Autodesk Inventor part; units mm, degrees
ref_plane "YZ Plane" through (0, 0, 0) normal (1, 0, 0) x (0, 1, 0)
ref_plane "XZ Plane" through (0, 0, 0) normal (0, 1, 0) x (-1, 0, 0)
ref_plane "XY Plane" through (0, 0, 0) normal (0, 0, 1) x (1, 0, 0)
sketch "Sketch1" plane through (0, 0, 0) normal (0, 0, 1) x (1, 0, 0)
  line L0 (-127.68, 259.036) -> (-127.68, -85.275)
  line L1 (-127.68, 259.036) -> (47.477, 259.036)
  line L2 (127.68, -259.036) -> (-32.32, -259.036)
  line L3 (-32.32, -259.036) -> (-127.68, -85.275)
  line L4 (127.68, -259.036) -> (127.68, -145.836)
  line L5 (127.68, -145.836) -> (47.477, 259.036)
  point P0 (0, 0)
  dimension "d6" = 344.311
  dimension "d7" = 175.157
  dimension "d9" = 160
  dimension "d10" = 113.2
extrude "Extrusion1" add sketch "Sketch1" along normal mid plane 13
sketch "Sketch2" plane through (0, 0, 6.5) normal (0, 0, 1) x (1, 0, 0)
  circle A0 centre (-71.723, 203.108) radius 9
  circle A1 centre (-71.723, 69.5056) radius 9
  line L0 (47.477, 259.036) -> (-127.68, 259.036)
  line L1 (-127.68, 259.036) -> (-127.68, -85.275)
  circle A2 centre (-71.723, 136.306) radius 5
  point P0 (0, 0)
  dimension "d17" = 55.957
  dimension "d39" = 10
  dimension "d43" = 55.928
  dimension "d44" = 66.8004
  dimension "d45" = 66.802
extrude "Extrusion4" cut sketch "Sketch2" against normal blind 25.4
properties part number "CNC-X-axis- side plates"
Can you work these out from the model? Positions are in its coordinate system, mm. Coordinates: 2 decimals unless noted, no trailing zeros. Loops run counter-clockwise (first coordinate to the right, second up) from the corner with the lowest first, then second, coordinate; pieces in that order, holes last. Notation, with made-up numbers: M -12,26.25 L 19,26.25 A19 cw 19,56.25 Z; hole C 48,30 d6. An arc over 180 degrees is marked long. Put each result on its own line as item: value. Start each with the question number.
(1) Will these pins go through, and if not, where does the flat tip stop? pin 1 Ø1 at (y, z) = (81, -4) entering from +X; pin 2 Ø16 at (x, y) = (-71.723, 203.108) entering from -Z.
(2) We'd pull the mould along X, two halves only. Please class faces 1 (the face through (88.14, 53.77, -0.09)), 2 (the face through (49, -259.036, 0)), 3 (the face through (-72.895, 212.031, 0.091)): +X half, -X half, draft (parallel to the pull), parting line (faces both ways), or undercut.
(3) Imagine slicing it at B-B on x = -109.5. List the corners of the cut face in (y, z) for me, and give its area (3 significant figures).
(4) Imagine slicing it at A-A on z = -1.5. List the corners of the cut face in (x, y) for me (3 decimals), and give its area (3 significant figures).
(5) I need wall thicknesses on probe 1 along X at (y, z) = (135.5, 3.5); probe 2 along X at (y, z) = (63.5, -3); probe 3 along X at (y, z) = (6, -5.25). Which ranges of each line are inside material? Lowest first, please.
(6) Imagine slicing it at C-C on y = -210. List the corners of the cut face in (x, z) for me.
Worked answers:
1. pin 1: stops at x = 82.84
1. pin 2: passes through
2. face 1: +X half
2. face 2: draft
2. face 3: undercut
3. outline: M -118.4,-6.5 L 259.04,-6.5 L 259.04,6.5 L -118.4,6.5 Z
3. area: 4,910 mm2
4. outline: M -127.68,-85.275 L -32.32,-259.036 L 127.68,-259.036 L 127.68,-145.836 L 47.477,259.036 L -127.68,259.036 Z; hole C -71.723,69.506 d18; hole C -71.723,203.108 d18; hole C -71.723,136.306 d10
4. area: 107,000 mm2
5. probe 1: x = -127.68 to -76.66, -66.79 to 71.95
5. probe 2: x = -127.68 to -78.43, -65.02 to 86.21
5. probe 3: x = -127.68 to 97.6
6. outline: M -59.23,-6.5 L 127.68,-6.5 L 127.68,6.5 L -59.23,6.5 Z
